Input: part model. Units: mm. Frame: model coordinates. Face numbers are marked on the shaded views. A direction names the side the tool comes from. Coordinates: 2 decimals unless noted, no trailing zeros. Order: outer loops, then holes, each group sorted by start corner. A loop starts at its lowest first (then second) coordinate and runs counter-clockwise, first axis right, second up. Notation, with made-up numbers: (-2, 10.5) - (7, 10.5) arc R31 ccw to (7, 36.5) - close; hole circle Ø6 at (25, 79.25). An arc over 180 degrees is marked (long way). One line per question, with ' | ' between items.
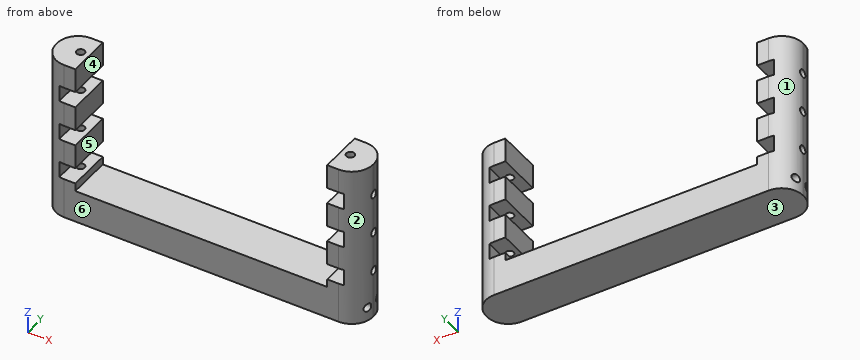
from build123d import *

# Parameters (mm, degrees)
F0_W         = 195
F0_H         = 100
F1_DEPTH     = 27
F2_W         = 155
F2_H         = 80
F3_DEPTH     = 27.001
F4_W         = 10
F4_H         = 10
F5_DEPTH     = 27.001
F6_R         = 2.5
F7_DEPTH     = 80
F9_DEPTH     = 195.001
F10_R        = 2.5
F11_DEPTH    = 195.001
F12_T1_DEPTH = 165


# Not quite as in the source:
# - a fillet or chamfer that OpenCascade refuses, or shapes differently, is made with other operations: its cross-section is extruded or revolved along the edge and cut away or added


with BuildPart() as f1:
    # F0 (on Front) → F1 (new body)
    with BuildSketch(Plane.XZ):
        with Locations((97.5, 50)):
            Rectangle(F0_W, F0_H)
    extrude(amount=F1_DEPTH)

    # F2 (on Front) → F3 (cut, through all)
    with BuildSketch(Plane.XZ):
        with Locations((97.5, 60)):
            Rectangle(F2_W, F2_H)
    extrude(amount=F3_DEPTH, mode=Mode.SUBTRACT)

    # F4 (on Front) → F5 (cut, through all)
    with BuildSketch(Plane.XZ):
        with Locations((180, 80)):
            Rectangle(F4_W, F4_H)
        with Locations((180, 55)):
            Rectangle(F4_W, F4_H)
        with Locations((180, 30)):
            Rectangle(F4_W, F4_H)
        with Locations((15, 30)):
            Rectangle(F4_W, F4_H)
        with Locations((15, 55)):
            Rectangle(F4_W, F4_H)
        with Locations((15, 80)):
            Rectangle(F4_W, F4_H)
    extrude(amount=F5_DEPTH, mode=Mode.SUBTRACT)

    # F6 (on face) → F7 (cut)
    with BuildSketch(Plane.XY.offset(100)):
        with Locations((180.5, -13)):
            Circle(F6_R)
        with Locations((14.5, -13)):
            Circle(F6_R)
    extrude(amount=-F7_DEPTH, mode=Mode.SUBTRACT)

    # F8 (on Right) → F9 (cut, through all)
    with BuildSketch(Plane.YZ):
        with BuildLine():
            Line((-13, 77.5), (-13, 82.5))
            ThreePointArc((-13, 82.5), (-15.5, 80), (-13, 77.5))
        make_face()
        with BuildLine():
            ThreePointArc((-13, 77.5), (-11.232233047, 78.232233047), (-10.5, 80))
            ThreePointArc((-10.5, 80), (-11.232233047, 81.767766953), (-13, 82.5))
            Line((-13, 82.5), (-13, 77.5))
        make_face()
        with BuildLine():
            Line((-13, 52.5), (-13, 57.5))
            ThreePointArc((-13, 57.5), (-15.5, 55), (-13, 52.5))
        make_face()
        with BuildLine():
            ThreePointArc((-10.5, 55), (-11.232233047, 56.767766953), (-13, 57.5))
            Line((-13, 57.5), (-13, 52.5))
            ThreePointArc((-13, 52.5), (-11.232233047, 53.232233047), (-10.5, 55))
        make_face()
        with BuildLine():
            Line((-13, 27.5), (-13, 32.5))
            ThreePointArc((-13, 32.5), (-15.5, 30), (-13, 27.5))
        make_face()
        with BuildLine():
            ThreePointArc((-10.5, 30), (-11.232233047, 31.767766953), (-13, 32.5))
            Line((-13, 32.5), (-13, 27.5))
            ThreePointArc((-13, 27.5), (-11.232233047, 28.232233047), (-10.5, 30))
        make_face()
    extrude(amount=F9_DEPTH, mode=Mode.SUBTRACT)

    # F10 (on Right) → F11 (cut, through all)
    with BuildSketch(Plane.YZ):
        with Locations((-8, 8.5)):
            Circle(F10_R)
        with Locations((-18, 8.5)):
            Circle(F10_R)
    extrude(amount=F11_DEPTH, mode=Mode.SUBTRACT)

    # F12: fillet of radius 13 on 4 edges, made by hand

    # F12_s2 → F12_t1 (cut)
    with BuildSketch(Plane.XY.offset(-32.5)):
        with BuildLine():
            ThreePointArc((0, -13), (3.8076118446, -3.8076118446), (13, 0))
            Line((13, 0), (0, 0))
            Line((0, 0), (0, -13))
        make_face()
        with BuildLine():
            ThreePointArc((0, -14), (3.8076118446, -23.1923881554), (13, -27))
            Line((13, -27), (0, -27))
            Line((0, -27), (0, -14))
        make_face()
        with BuildLine():
            ThreePointArc((182, -27), (191.1923881554, -23.1923881554), (195, -14))
            Line((195, -14), (195, -27))
            Line((195, -27), (182, -27))
        make_face()
        with BuildLine():
            ThreePointArc((182, 0), (191.1923881554, -3.8076118446), (195, -13))
            Line((195, -13), (195, 0))
            Line((195, 0), (182, 0))
        make_face()
    extrude(amount=F12_T1_DEPTH, mode=Mode.SUBTRACT)


solid = f1.part
Item 1: Section B-B on x = 127. Return the cut outline in (y, z).
Data:
outline: (-27, 0) - (0, 0) - (0, 20) - (-27, 20) - close; hole circle Ø5 at (-18, 8.5); hole circle Ø5 at (-8, 8.5)
Item 2: Draft query along X for the marked faces 1, 2, 3 and 4. Return one class per face: released by +X, released by -X, zero draft, split by the parting line, or undercut.
Data:
face 1: released by -X | face 2: released by +X | face 3: zero draft | face 4: undercut
Item 3: Access query for the marked faces 5 and 6. Directions: +Z, -Z, +X, -X, +Y, -Y. A direction counts if a zero-diameter tool reaches every point of the face in a straight line with its end or side. Return the directions, or none.
Data:
face 5: +Z, +Y, -Y | face 6: +Z, -Z, +X, -X, -Y
Item 4: Contact query for flat-ended pins moving along their axis: P1, Ø8, axis at y = -20, z = 44, coming from the +X side; P2, Ø3, axis at y = -8, z = 8.5, coming from the +X side; P3, Ø4.5, axis at y = -19, z = 91.5, coming from the -X side; P4, Ø3, axis at y = -18.5, z = 28.5, coming from the -X side. Output: stop coordinate, or through.
Data:
P1: x = 194.85 | P2: through | P3: x = 0.29 | P4: x = 0.35
Item 5: Section A-A on z = 92. Return the cut outline in (x, y).
Data:
outline: (0, -14) arc R13 ccw to (13, -27) - (20, -27) - (20, 0) - (13, 0) arc R13 ccw to (0, -13) - close; (175, -27) - (182, -27) arc R13 ccw to (195, -14) - (195, -13) arc R13 ccw to (182, 0) - (175, 0) - close; hole circle Ø5 at (14.5, -13); hole circle Ø5 at (180.5, -13)
Item 6: Ray query, line 1 (Y direction, x = 14.5, z = 38.25); line 2 (Z direction, x = 53, y = -14.25); line 3 (Z direction, x = 87.5, y = -7.25). Return the intervals inside material, ascending.
Data:
line 1: -27 to -15.5, -10.5 to 0 | line 2: 0 to 20 | line 3: 0 to 6.12, 10.88 to 20
